```python
from build123d import *

# Parameters (mm, degrees)
SKETCH1_W           = 660.4
SKETCH1_H           = 660.4
SKETCH1_W_2         = 609.6
SKETCH1_H_2         = 609.6
BOSS_EXTRUDE1_DEPTH = 50.8
SKETCH2_W           = 660.4
SKETCH2_H           = 50.8
BOSS_EXTRUDE2_DEPTH = 25.4
SKETCH3_W           = 25.4
SKETCH3_H           = 50.8
BOSS_EXTRUDE3_DEPTH = 939.8
BOSS_EXTRUDE4_START = 73.025
SKETCH4_R           = 6.35
BOSS_EXTRUDE4_DEPTH = 133.35
SKETCH4_2_R         = 6.35
BOSS_EXTRUDE5_DEPTH = 282.956
SKETCH5_W           = 825.5
SKETCH5_H           = 825.5
SKETCH5_W_2         = 660.4
SKETCH5_H_2         = 660.4
BOSS_EXTRUDE6_DEPTH = 76.2


with BuildPart() as part:
    # Sketch1 → Boss-Extrude1 (new body)
    with BuildSketch(Plane.XY):
        with Locations((330.2, 330.2)):
            Rectangle(SKETCH1_W, SKETCH1_H)
        with Locations((330.2, 330.2)):
            Rectangle(SKETCH1_W_2, SKETCH1_H_2, mode=Mode.SUBTRACT)
    extrude(amount=BOSS_EXTRUDE1_DEPTH)

    # Sketch2 → Boss-Extrude2 (add)
    with BuildSketch(Plane.XY.offset(50.8)):
        with Locations((330.2, 292.1)):
            Rectangle(SKETCH2_W, SKETCH2_H)
    extrude(amount=BOSS_EXTRUDE2_DEPTH)

    # Sketch3 → Boss-Extrude3 (add)
    with BuildSketch(Plane.XY.offset(76.2)):
        with Locations((177.8, 292.1)):
            Rectangle(SKETCH3_W, SKETCH3_H)
        with Locations((482.6, 292.1)):
            Rectangle(SKETCH3_W, SKETCH3_H)
    extrude(amount=BOSS_EXTRUDE3_DEPTH)



with BuildPart() as body_2:
    # Sketch4 → Boss-Extrude4 (new body)
    with BuildSketch(Plane.ZY.offset(-469.9).offset(BOSS_EXTRUDE4_START)):
        Polygon((485.515641783, 358.684996296), (310.689543984, 109.007453196), (352.302467833, 79.86977023), (596.712759729, -9.088300969), (771.538857529, 240.589242131), (527.128565633, 329.547313329), align=None)
        with Locations((469.9, 292.1)):
            Circle(SKETCH4_R, mode=Mode.SUBTRACT)
    extrude(amount=BOSS_EXTRUDE4_DEPTH)


with BuildPart() as part_1:
    add(part.part)

    add(body_2.part)  # Boss-Extrude5 merges body 2
    # Sketch4<2> → Boss-Extrude5 (add)
    with BuildSketch(Plane.ZY.offset(-469.9)):
        with Locations((469.9, 292.1)):
            Circle(SKETCH4_2_R)
    extrude(amount=BOSS_EXTRUDE5_DEPTH)

    # Sketch5 → Boss-Extrude6 (add)
    with BuildSketch(Plane.XY):
        with Locations((330.2, 330.2)):
            Rectangle(SKETCH5_W, SKETCH5_H)
        with Locations((330.2, 330.2)):
            Rectangle(SKETCH5_W_2, SKETCH5_H_2, mode=Mode.SUBTRACT)
    extrude(amount=BOSS_EXTRUDE6_DEPTH)


solid = part_1.part
```
Could you check a few things on this model? Use its own coordinates, in mm. A direction names the side the tool comes from. Round coordinates to 2 decimals unless told otherwise and drop trailing zeros. Order: outer loops, then holes, each group sorted by start corner. A loop starts at its lowest first (then second) coordinate and runs counter-clockwise, first axis right, second up. Notation, with made-up numbers: M 67,-3 L 81,-3 A19 ccw 81,4 Z; hole C 43.25,-30.75 d8. An arc over 180 degrees is marked long. One line per question, with ' | ' between items. Start each with the question number.
(1) For faces 5 (the face through (0, 131, 63)), 6 (the face through (326, 635, 25)), 7 (the face through (329, 15, 50.8)), which set-ups out of +Z, -Z, +X, -X, +Y, -Y let a thin tool reach every point of the face, with its end or its side?
(2) Suppose I cut it at C-C on z = 841. List the corners of the cut face in (x, y) for me.
(3) Thinking about a two-plate mould opening in Y: for faces 1 (the face through (475, 317.5, 388)), 2 (the face through (190.5, 292, 540)), 3 (the face through (324, -82.55, 38)), 4 (the face through (326, 0, 63)), which applies, +Y half, -Y half, draft (parallel to the pull), parting line (faces both ways), or undercut?
(4) Please list where these lines run through material, in increasing order: line 1 along Y through (x, z) = (170.5, 291); line 2 along Z through (x, y) = (648, 89.5); line 3 along X through (y, z) = (148.5, 402) (3 decimals).
(5) For P1, Ø2, axis at x = 554, y = 287.5, coming from the +Z side; P2, Ø8, axis at x = 282.5, z = 590.5, coming from the +Y side; P3, Ø15, axis at y = 286, z = 364.5, coming from the -X side, each with a flat end and sliding along its axis, tell me the tip position at first contact or that it passes through.
(6) Suppose I cut it at A-A on x = 145.5. List the corners of the cut face in (y, z) for me, then the cut area to 3 significant figures.
(7) Suppose I cut it at B-B on y = 477. List the corners of the cut face in (x, z) for me.
(8) Suppose I cut it at D-D on x = 344. List the corners of the cut face in (y, z) for me (3 decimals), then the cut area to 3 significant figures.
Geometry results:
1) face 5: +Z | face 6: +Z, -Z | face 7: none
2) outline: M 165.1,266.7 L 190.5,266.7 L 190.5,317.5 L 165.1,317.5 Z; M 469.9,266.7 L 495.3,266.7 L 495.3,317.5 L 469.9,317.5 Z
3) face 1: undercut | face 2: draft | face 3: -Y half | face 4: undercut
4) line 1: 266.7 to 317.5 | line 2: 0 to 50.8 | line 3: 263.525 to 396.875
5) P1: z = 76.2 | P2: y = 307.94 | P3: x = 165.1
6) outline: M -82.55,0 L 25.4,0 L 25.4,50.8 L 0,50.8 L 0,76.2 L -82.55,76.2 Z; M 266.7,50.8 L 317.5,50.8 L 317.5,76.2 L 266.7,76.2 Z; M 635,0 L 742.95,0 L 742.95,76.2 L 660.4,76.2 L 660.4,50.8 L 635,50.8 Z | area: 16,500 mm²
7) outline: M -82.55,0 L 25.4,0 L 25.4,50.8 L 0,50.8 L 0,76.2 L -82.55,76.2 Z; M 635,0 L 742.95,0 L 742.95,76.2 L 660.4,76.2 L 660.4,50.8 L 635,50.8 Z
8) outline: M -82.55,0 L 25.4,0 L 25.4,50.8 L 0,50.8 L 0,76.2 L -82.55,76.2 Z; M -9.088,596.713 L 79.87,352.302 L 109.007,310.69 L 358.685,485.516 L 329.547,527.129 L 240.589,771.539 Z; M 266.7,50.8 L 317.5,50.8 L 317.5,76.2 L 266.7,76.2 Z; M 635,0 L 742.95,0 L 742.95,76.2 L 660.4,76.2 L 660.4,50.8 L 635,50.8 Z | area: 109,000 mm²
